```python
from build123d import *

# Parameters (mm, degrees)
SKETCH1_R           = 21.5
BOSS_EXTRUDE1_DEPTH = 30
SKETCH2_R           = 18
CUT_EXTRUDE1_DEPTH  = 25
SKETCH4_R           = 10.5
CUT_EXTRUDE2_DEPTH  = 43.714166268
FILLET1_R           = 3
SKETCH5_W           = 1
SKETCH5_H           = 0.5
CHAMFER1_SIZE       = 4
CHAMFER1_SIZE2      = 1.455880937


with BuildPart() as part:
    # Sketch1 → Boss-Extrude1 (new body)
    with BuildSketch(Plane(origin=(0, 0, 0), x_dir=(0, 0, -1), z_dir=(1, 0, 0))):
        Circle(SKETCH1_R)
    extrude(amount=BOSS_EXTRUDE1_DEPTH)

    # Sketch2 → Cut-Extrude1 (cut)
    with BuildSketch(Plane(origin=(30, 0, 0), x_dir=(0, 0, -1), z_dir=(1, 0, 0))):
        Circle(SKETCH2_R)
    extrude(amount=-CUT_EXTRUDE1_DEPTH, mode=Mode.SUBTRACT)

    # Sketch4 → Cut-Extrude2 (cut, through all)
    with BuildSketch(Plane.ZY):
        Circle(SKETCH4_R)
    extrude(amount=-CUT_EXTRUDE2_DEPTH, mode=Mode.SUBTRACT)

    # Fillet1
    fillet1_edges = [part.edges().sort_by_distance(p)[0] for p in [
        (0, 0, 21.5),
        (30, 0, 21.5),
    ]]
    fillet(fillet1_edges, radius=FILLET1_R)

    # Sketch5 → Cut-Revolve1 (revolve, cut)
    with BuildSketch(Plane.XY, mode=Mode.PRIVATE) as cut_revolve1_sk:
        with Locations((5.5, 21.25)):
            Rectangle(SKETCH5_W, SKETCH5_H)
        with Locations((24.5, 21.25)):
            Rectangle(SKETCH5_W, SKETCH5_H)
        with Locations((10.5, 21.25)):
            Rectangle(SKETCH5_W, SKETCH5_H)
        with Locations((19.5, 21.25)):
            Rectangle(SKETCH5_W, SKETCH5_H)
    revolve(cut_revolve1_sk.sketch.rotate(Axis((0, 0, 0), (1, 0, 0)), 90), axis=Axis((0, 0, 0), (1, 0, 0)), mode=Mode.SUBTRACT)

    # Chamfer1
    chamfer1_edges = [part.edges().sort_by_distance(p)[0] for p in [
        (5, 0, 18),
    ]]
    chamfer1_side = [part.faces().sort_by_distance(p)[0] for p in [
        (17.5, 0, 18),
    ]]
    chamfer(chamfer1_edges, length=CHAMFER1_SIZE, length2=CHAMFER1_SIZE2, reference=chamfer1_side[0])


solid = part.part
```
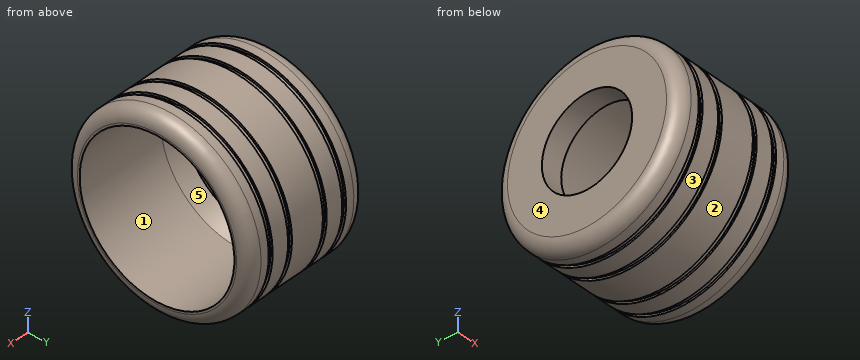
CAD build for the part. Positions are in the model's coordinates, mm. Face numbers are marked on the shaded views. A direction names the side the tool comes from. Round coordinates to 2 decimals unless told otherwise and drop trailing zeros. Order: outer loops, then holes, each group sorted by start corner. A loop starts at its lowest first (then second) coordinate and runs counter-clockwise, first axis right, second up. Notation, with made-up numbers: (82, -14) - (105, -14) arc R25 cw to (105, -2) - close; hole circle Ø8 at (87, -22). An arc over 180 degrees is marked (long way). Answer as CSV lines item,"result". Start each with the question number.
1. Drill centre lines: L1, parallel to Y at x = 3.35, z = 0; L2, parallel to Y at x = 15.25, z = 0; L3, parallel to X at y = 10, z = 10. Where is each one in solid material? Low to high. Write a range as [from, to].
2. Saw through at B-B, the plane x = 6.75. Write the cut outline in (y, z), and give its area (3 significant figures).
3. Pull direction Y, two halves, no side cores. Call the marked faces 3, 4 and 5: +Y half, -Y half, draft (parallel to the pull), parting line (faces both ways), or undercut.
4. Tool access for the marked faces 1 and 2: list every direction of +Z, -Z, +X, -X, +Y, -Y with a clear straight run to the whole face (end or side of a thin tool).
5. Saw through at A-A, the plane x = 22.25. Write the cut outline in (y, z).
6. Pin check, flat tips, straight feed: pin 1 (13 mm diameter, centred on y = -2.5, z = -1, fed in from +X); pin 2 (8 mm diameter, centred on x = 24, z = -11.5, fed in from -Y); pin 3 (6 mm diameter, centred on x = 11, y = -15.5, fed in from +Z); pin 4 (12 mm diameter, centred on x = 14, y = 7, fed in from +Z). Stop position of each tip, or through.
Model answer:
1,L1,"y = [-21.5, -10.5], [10.5, 21.5]"
1,L2,"y = [-21.5, -18], [18, 21.5]"
1,L3,"x = [0, 5]"
2,outline,"circle Ø43 at (0, 0); hole circle Ø34.36 at (0, 0)"
2,area,"525 mm²"
3,face 3,"parting line"
3,face 4,"draft"
3,face 5,"undercut"
4,face 1,"+X"
4,face 2,"+X, -X"
5,outline,"circle Ø43 at (0, 0); hole circle Ø36 at (0, 0)"
6,pin 1,"passes through"
6,pin 2,"stops at y = -20.15"
6,pin 3,"stops at z = 17.49"
6,pin 4,"stops at z = 21.48"
